Work out the finished part from the listing and answer in its coordinate system (mm). Face numbers are marked on the shaded views. A direction names the side the tool comes from. Round coordinates to 2 decimals unless told otherwise and drop trailing zeros. Write each loop counter-clockwise with the first axis right and the second up, starting at its lowest first coordinate (ties: lowest second). Pieces come first, ordered by that corner, then holes.
1. A tool of negligible diameter and unlimited length cuts with its end or side. For the marked faces 1, 2 and 3, from which of +Z, -Z, +X, -X, +Y, -Y can it reach the whole face along a straight path? Write none if from no direction.
2. Straight lines are drawn through the part: probe 1 along X at (y, z) = (-8.25, 25.5); probe 2 along Y at (x, z) = (22, 15); probe 3 along X at (y, z) = (8.75, 1.75). For each, find the intervals that lie inside material, in ascending order.
3. Find section C-C (y = 8.5). Write down the section's boundary in (x, z).
4. Flat-ended cylindrical pins translate along their axes: pin 1 Ø1.4 at (x, z) = (9.35, 3.5) entering from -Y; pin 2 Ø2 at (y, z) = (2.5, 17.5) entering from -X; pin 3 Ø3 at (x, z) = (5, 13) entering from +Y. Find the tip coordinate at first contact, or state that the pin passes through.
5. Find section D-D (x = 4.5). Write down the section's boundary in (y, z), and give its area (3 significant figures).
6. Determine the mould class of the marked faces 4, 5 and 6 for opening direction X: pulls with the +X half, pulls with the -X half, needs draft (parallel to the pull), parting line crosses it, or undercut.
7. Find section A-A (z = 15). Write down the section's boundary in (x, y).
8. Find section B-B (z = 3.5). Write down the section's boundary in (x, y).
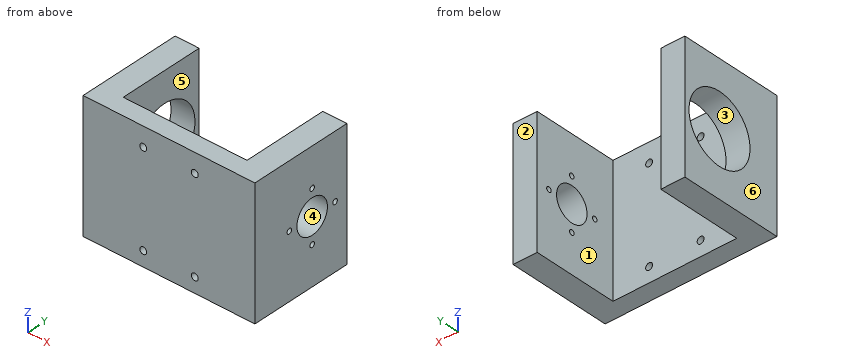
```python
from build123d import *

# Parameters (mm, degrees)
SKETCH1_W                 = 40.0059906
SKETCH1_H                 = 24.13
BOSS_EXTRUDE1_DEPTH       = 30
SKETCH6_W                 = 28.8299906
SKETCH6_H                 = 19.896666666
CUT_EXTRUDE1_DEPTH        = 30
SKETCH9_R                 = 0.8
CUT_EXTRUDE3_DEPTH        = 30
SKETCH29_R                = 8.001
CUT_EXTRUDE4_DEPTH        = 5.588
SKETCH41_R                = 4
CUT_EXTRUDE5_DEPTH        = 5.588
F_0_80_TAPPED_HOLE1_D     = 1.19126
F_0_80_TAPPED_HOLE1_DEPTH = 5.588


with BuildPart() as part:
    # Sketch1 → Boss-Extrude1 (new body)
    with BuildSketch(Plane.XY):
        with Locations((3.348789693, 2.822850467)):
            Rectangle(SKETCH1_W, SKETCH1_H)
    extrude(amount=BOSS_EXTRUDE1_DEPTH)

    # Sketch6 → Cut-Extrude1 (cut)
    with BuildSketch(Plane.XY.offset(30)):
        with Locations((3.348789693, 4.939517134)):
            Rectangle(SKETCH6_W, SKETCH6_H)
    extrude(amount=-CUT_EXTRUDE1_DEPTH, mode=Mode.SUBTRACT)

    # Sketch9 → Cut-Extrude3 (cut)
    with BuildSketch(Plane(origin=(0, -9.242149533, 0), x_dir=(-1, 0, 0), z_dir=(0, -1, 0))):
        with Locations((2.651210307, -25.5)):
            Circle(SKETCH9_R)
        with Locations((-9.348789693, -25.5)):
            Circle(SKETCH9_R)
        with Locations((-9.348789693, -3.5)):
            Circle(SKETCH9_R)
        with Locations((2.651210307, -3.5)):
            Circle(SKETCH9_R)
    extrude(amount=-CUT_EXTRUDE3_DEPTH, mode=Mode.SUBTRACT)

    # Sketch29 → Cut-Extrude4 (cut)
    with BuildSketch(Plane.ZY.offset(16.654205607)):
        with Locations((15, 5.794650467)):
            Circle(SKETCH29_R)
    extrude(amount=-CUT_EXTRUDE4_DEPTH, mode=Mode.SUBTRACT)

    # Sketch41 → Cut-Extrude5 (cut)
    with BuildSketch(Plane(origin=(23.351784993, 0, 0), x_dir=(0, 0, -1), z_dir=(1, 0, 0))):
        with Locations((-15, 5.794650467)):
            Circle(SKETCH41_R)
    extrude(amount=-CUT_EXTRUDE5_DEPTH, mode=Mode.SUBTRACT)

    # #0-80 Tapped Hole1
    with Locations(Plane(origin=(23.351784993, 0, 0), x_dir=(0, 0, -1), z_dir=(1, 0, 0))):
        with Locations((-15, 11.794650467), (-9, 5.794650467), (-15, -0.205349533), (-21, 5.794650467)):
            Hole(F_0_80_TAPPED_HOLE1_D / 2, depth=F_0_80_TAPPED_HOLE1_DEPTH)


solid = part.part
```
Worked answers:
1. face 1: +Z, -Z, +Y
1. face 2: +Z, -Z, +X, -X, +Y
1. face 3: -X
2. probe 1: x = -16.65 to -3.45, -1.85 to 8.55, 10.15 to 23.35
2. probe 2: y = -9.24 to -0.8, 0.39 to 1.79, 9.79 to 11.2, 12.39 to 14.89
2. probe 3: x = -16.65 to -11.07, 17.76 to 23.35
3. outline: (-16.65, 0) - (-11.07, 0) - (-11.07, 7.47) - (-16.65, 7.47) - close; (-16.65, 22.53) - (-11.07, 22.53) - (-11.07, 30) - (-16.65, 30) - close; (17.76, 0) - (23.35, 0) - (23.35, 12.05) - (17.76, 12.05) - close; (17.76, 17.95) - (23.35, 17.95) - (23.35, 30) - (17.76, 30) - close
4. pin 1: passes through
4. pin 2: stops at x = 17.76
4. pin 3: stops at y = -5.01
5. outline: (-9.24, 0) - (-5.01, 0) - (-5.01, 30) - (-9.24, 30) - close
5. area: 127 mm2
6. face 4: needs draft
6. face 5: undercut
6. face 6: pulls with the -X half
7. outline: (-16.65, -9.24) - (23.35, -9.24) - (23.35, -0.8) - (17.76, -0.8) - (17.76, -5.01) - (-11.07, -5.01) - (-11.07, -2.21) - (-16.65, -2.21) - close; (-16.65, 13.8) - (-11.07, 13.8) - (-11.07, 14.89) - (-16.65, 14.89) - close; (17.76, 0.39) - (23.35, 0.39) - (23.35, 1.79) - (17.76, 1.79) - close; (17.76, 9.79) - (23.35, 9.79) - (23.35, 11.2) - (17.76, 11.2) - close; (17.76, 12.39) - (23.35, 12.39) - (23.35, 14.89) - (17.76, 14.89) - close
8. outline: (-16.65, -9.24) - (-3.45, -9.24) - (-3.45, -5.01) - (-11.07, -5.01) - (-11.07, 14.89) - (-16.65, 14.89) - close; (-1.85, -9.24) - (8.55, -9.24) - (8.55, -5.01) - (-1.85, -5.01) - close; (10.15, -9.24) - (23.35, -9.24) - (23.35, 14.89) - (17.76, 14.89) - (17.76, -5.01) - (10.15, -5.01) - close
